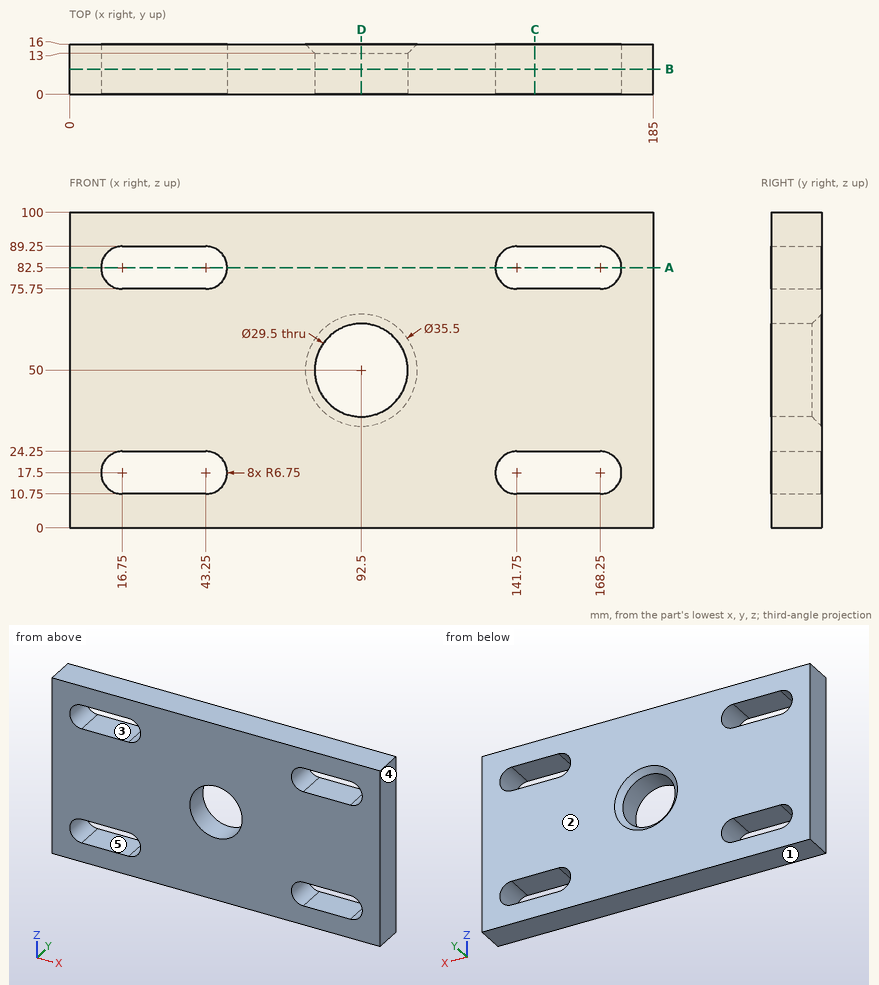
Answer from the drawing. Dimensions are ordinates in mm from the lowest x, y and z of the part. A direction names the side the tool comes from. Coordinates: 2 decimals unless noted, no trailing zeros. Write each loop counter-clockwise with the first axis right and the second up, starting at its lowest first coordinate (ties: lowest second). Pieces come first, ordered by that corner, then holes. Notation, with made-up numbers: (72.25, 68.25) - (97.25, 68.25) arc R15 ccw to (97.25, 75.25) - close; hole circle Ø9 at (54.25, 11.5). An arc over 180 degrees is marked (long way). One line per question, with ' | ' between items.
Q1. Find section D-D, the plane x = 92.5. Write down the section's boundary in (y, z).
Result set:
outline: (0, 0) - (16, 0) - (16, 32.25) - (13, 35.25) - (0, 35.25) - close; (0, 64.75) - (13, 64.75) - (16, 67.75) - (16, 100) - (0, 100) - close
Q2. Consider L1, parallel to Z at x = 25.5, y = 14.5; L2, parallel to X at y = 5.25, z = 50; L3, parallel to X at y = 10, z = 12.5. Determine where each line is inside the solid, lowest interval first. Write a range as [from, to].
Result set:
L1: [0, 10.75], [24.25, 75.75], [89.25, 100] | L2: [0, 77.75], [107.25, 185] | L3: [0, 12.22], [47.78, 137.22], [172.78, 185]
Q3. Find section B-B, the plane y = 8. Write down the section's boundary in (x, z).
Result set:
outline: (0, 0) - (185, 0) - (185, 100) - (0, 100) - close; hole (16.75, 10.75) - (43.25, 10.75) arc R6.75 ccw to (43.25, 24.25) - (16.75, 24.25) arc R6.75 ccw to start; hole (16.75, 75.75) - (43.25, 75.75) arc R6.75 ccw to (43.25, 89.25) - (16.75, 89.25) arc R6.75 ccw to start; hole circle Ø29.5 at (92.5, 50); hole (141.75, 10.75) - (168.25, 10.75) arc R6.75 ccw to (168.25, 24.25) - (141.75, 24.25) arc R6.75 ccw to start; hole (141.75, 75.75) - (168.25, 75.75) arc R6.75 ccw to (168.25, 89.25) - (141.75, 89.25) arc R6.75 ccw to start
Q4. Find section A-A, the plane z = 82.5. Write down the section's boundary in (x, y).
Result set:
outline: (0, 0) - (10, 0) - (10, 16) - (0, 16) - close; (50, 0) - (135, 0) - (135, 16) - (50, 16) - close; (175, 0) - (185, 0) - (185, 16) - (175, 16) - close
Q5. Determine the mould class of the marked faces 1, 2 and 3 for opening direction Z: +Z half, -Z half, draft (parallel to the pull), parting line (faces both ways), or undercut.
Result set:
face 1: -Z half | face 2: draft | face 3: undercut
Q6. For the marked faces 4 and 5, determine the directions among +Z, -Z, +X, -X, +Y, -Y from which every point of the face is accessible in a straight line to the end or side of a thin tool.
Result set:
face 4: +Z, -Z, +X, +Y, -Y | face 5: +Y, -Y
Q7. This flat-tipped pin is pushed along its axis until it touches: P1, Ø3, axis at x = 91, z = 25, coming from the -Y side. Where does it stop, or does it pass through?
Result set:
P1: y = 0
Q8. Find section C-C, the plane x = 147.5. Write down the section's boundary in (y, z).
Result set:
outline: (0, 0) - (16, 0) - (16, 10.75) - (0, 10.75) - close; (0, 24.25) - (16, 24.25) - (16, 75.75) - (0, 75.75) - close; (0, 89.25) - (16, 89.25) - (16, 100) - (0, 100) - close
